from build123d import *

# Parameters (mm, degrees)
SKETCH1_R                      = 27.5
SKETCH1_R_2                    = 8.05
BOSS_EXTRUDE1_DEPTH            = 10
SKETCH1_4_R                    = 3.05
CUT_EXTRUDE1_DEPTH             = 4
CBORE_FOR_M4_SHCS1_D           = 4.1
CBORE_FOR_M4_SHCS1_CBORE_D     = 8
CBORE_FOR_M4_SHCS1_CBORE_DEPTH = 4
CIRPATTERN1_COUNT              = 6
SKETCH1_5_R                    = 9.05
CUT_EXTRUDE2_DEPTH             = 8
BOSS_EXTRUDE2_START            = 8
SKETCH1_6_R                    = 29.5
SKETCH1_6_R_2                  = 27.5
BOSS_EXTRUDE2_DEPTH            = 2
M5X0_8_TAPPED_HOLE1_D          = 4.2
CBORE_FOR_M3_SHCS1_D           = 3.4
CBORE_FOR_M3_SHCS1_CBORE_D     = 6.5
CBORE_FOR_M3_SHCS1_CBORE_DEPTH = 3
CIRPATTERN2_COUNT              = 6
SKETCH9_R                      = 11
CUT_EXTRUDE3_DEPTH             = 4


with BuildPart() as part:
    # Sketch1 → Boss-Extrude1 (new body)
    with BuildSketch(Plane(origin=(0, 0, 0), x_dir=(1, 0, 0), z_dir=(0, 1, 0))):
        with Locations(Location((0, 0, 0), (0, 0, 270))):
            Circle(SKETCH1_R)
        with Locations(Location((0, 0, 0), (0, 0, 270))):
            Circle(SKETCH1_R_2, mode=Mode.SUBTRACT)
    extrude(amount=BOSS_EXTRUDE1_DEPTH)

    # Sketch1<4> → Cut-Extrude1 (cut)
    with BuildSketch(Plane(origin=(0, 0, 0), x_dir=(1, 0, 0), z_dir=(0, 1, 0))):
        with Locations(Location((-20, 0, 0), (0, 0, 270))):
            Circle(SKETCH1_4_R)
        with Locations(Location((-10, 17.320508076, 0), (0, 0, 270))):
            Circle(SKETCH1_4_R)
        with Locations(Location((10, 17.320508076, 0), (0, 0, 270))):
            Circle(SKETCH1_4_R)
        with Locations(Location((20, 0, 0), (0, 0, 270))):
            Circle(SKETCH1_4_R)
        with Locations(Location((10, -17.320508076, 0), (0, 0, 270))):
            Circle(SKETCH1_4_R)
        with Locations(Location((-10, -17.320508076, 0), (0, 0, 270))):
            Circle(SKETCH1_4_R)
    extrude(amount=CUT_EXTRUDE1_DEPTH, mode=Mode.SUBTRACT)

    # CBORE for M4 SHCS1 (through all)
    with Locations(Plane(origin=(0, 10, 0), x_dir=(1, 0, 0), z_dir=(0, 1, 0))):
        with Locations((-20, 0)):
            cbore_for_m4_shcs1 = CounterBoreHole(CBORE_FOR_M4_SHCS1_D / 2, CBORE_FOR_M4_SHCS1_CBORE_D / 2, CBORE_FOR_M4_SHCS1_CBORE_DEPTH)

    # CirPattern1: CBORE for M4 SHCS1 ×6 about axis
    cirpattern1_axis = Axis((0, 0, 0), (0, 1, 0))
    for i in range(1, CIRPATTERN1_COUNT):
        add(cbore_for_m4_shcs1.rotate(cirpattern1_axis, i * 360 / CIRPATTERN1_COUNT), mode=Mode.SUBTRACT)

    # Sketch1<5> → Cut-Extrude2 (cut)
    with BuildSketch(Plane(origin=(0, 0, 0), x_dir=(1, 0, 0), z_dir=(0, 1, 0))):
        with Locations(Location((0, 0, 0), (0, 0, 270))):
            Circle(SKETCH1_5_R)
    extrude(amount=CUT_EXTRUDE2_DEPTH, mode=Mode.SUBTRACT)

    # Sketch1<6> → Boss-Extrude2 (add)
    with BuildSketch(Plane(origin=(0, 0, 0), x_dir=(1, 0, 0), z_dir=(0, 1, 0)).offset(BOSS_EXTRUDE2_START)):
        with Locations(Location((0, 0, 0), (0, 0, 270))):
            Circle(SKETCH1_6_R)
        with Locations(Location((0, 0, 0), (0, 0, 270))):
            Circle(SKETCH1_6_R_2, mode=Mode.SUBTRACT)
    extrude(amount=BOSS_EXTRUDE2_DEPTH)

    # M5x0.8 Tapped Hole1 (through all)
    with Locations(Plane(origin=(0, 10, 0), x_dir=(1, 0, 0), z_dir=(0, 1, 0))):
        with Locations((0, 23)):
            m5x0_8_tapped_hole1 = Hole(M5X0_8_TAPPED_HOLE1_D / 2)

    # CBORE for M3 SHCS1 (through all)
    with Locations(Plane(origin=(0, 10, 0), x_dir=(1, 0, 0), z_dir=(0, 1, 0))):
        with Locations((0, 15)):
            cbore_for_m3_shcs1 = CounterBoreHole(CBORE_FOR_M3_SHCS1_D / 2, CBORE_FOR_M3_SHCS1_CBORE_D / 2, CBORE_FOR_M3_SHCS1_CBORE_DEPTH)

    # CirPattern2: M5x0.8 Tapped Hole1, CBORE for M3 SHCS1 ×6 about axis
    cirpattern2_axis = Axis((0, 0, 0), (0, 1, 0))
    add([m5x0_8_tapped_hole1.rotate(cirpattern2_axis, i * 360 / CIRPATTERN2_COUNT) for i in range(1, CIRPATTERN2_COUNT)], mode=Mode.SUBTRACT)
    add([cbore_for_m3_shcs1.rotate(cirpattern2_axis, i * 360 / CIRPATTERN2_COUNT) for i in range(1, CIRPATTERN2_COUNT)], mode=Mode.SUBTRACT)

    # Sketch9 → Cut-Extrude3 (cut)
    with BuildSketch(Plane.XZ):
        with Locations(Location((0, 0, 0), (0, 0, 270))):
            Circle(SKETCH9_R)
    extrude(amount=-CUT_EXTRUDE3_DEPTH, mode=Mode.SUBTRACT)


solid = part.part
Build history of the part. All positions in model axes, mm. A direction names the side the tool comes from. Coordinates: 2 decimals unless noted, no trailing zeros. Order: outer loops, then holes, each group sorted by start corner. A loop starts at its lowest first (then second) coordinate and runs counter-clockwise, first axis right, second up. Notation, with made-up numbers: (12.5, -4) - (38.5, -4) arc R23 cw to (38.5, 6) - close; hole circle Ø2 at (39, 68.25). An arc over 180 degrees is marked (long way). Write each question's results on one line, items separated by ' | '. Start each with the question number.
Item 1: Band-saw the part on C-C on y = 2. State how many separate pieces and enclosed holes the cut face has, and give its area (3 significant figures).
Item 2: Tool access for faces 1 (the face through (-13.36, 3.45, -9.16)), 2 (the face through (-9, 4, -2)), 3 (the face through (-22, 6, -1)): list every direction of +Z, -Z, +X, -X, +Y, -Y with a clear straight run to the whole face (end or side of a thin tool).
Item 3: Flat gauge pins, fed straight in: pin 1 (5 mm diameter, centred on x = -9.5, z = 18, fed in from -Y); pin 2 (6.5 mm diameter, centred on x = 10, z = 17.32, fed in from +Y); pin 3 (2 mm diameter, centred on x = 17.5, y = 5, fed in from -Z); pin 4 (1.5 mm diameter, centred on x = -5.5, y = 6, fed in from -Z). Where does each tip first touch, or does it go through?
Item 4: Band-saw the part on A-A on z = 23. Write the cut outline in (x, y).
Item 5: Band-saw the part on B-B on x = -20. Write the cut outline in (y, z).
Item 6: Wall check: probe 1 along X at (y, z) = (2.8, 0); probe 2 along Z at (x, y) = (-18.5, 7); probe 3 along Z at (x, y) = (-3, 9). Give the ranges that are in metal, low to high. Write a range as [from, to].
Numbers:
1) separate pieces: 1 | enclosed holes: 19 | area: 1,680 mm^2
2) face 1: +Y, -Y | face 2: -Y | face 3: +Y
3) pin 1: y = 0 | pin 2: y = 6 | pin 3: z = -22 | pin 4: z = -27.09
4) outline: (-18.47, 8) - (-15.07, 8) - (-15.07, 0) - (-2.1, 0) - (-2.1, 10) - (-18.47, 10) - close; (2.1, 0) - (15.07, 0) - (15.07, 8) - (18.47, 8) - (18.47, 10) - (2.1, 10) - close
5) outline: (0, -18.87) - (8, -18.87) - (8, -21.69) - (10, -21.69) - (10, -13.6) - (0, -13.6) - close; (0, -9.4) - (10, -9.4) - (10, -4) - (6, -4) - (6, -2.05) - (4, -2.05) - (4, -3.05) - (0, -3.05) - close; (0, 3.05) - (4, 3.05) - (4, 2.05) - (6, 2.05) - (6, 4) - (10, 4) - (10, 9.4) - (0, 9.4) - close; (0, 13.6) - (10, 13.6) - (10, 21.69) - (8, 21.69) - (8, 18.87) - (0, 18.87) - close
6) probe 1: [-27.5, -23.05], [-16.95, -11], [11, 16.95], [23.05, 27.5] | probe 2: [-20.35, -13.05], [-9.95, -3.71], [3.71, 9.95], [13.05, 20.35] | probe 3: [-29.35, -16.25], [-13.75, -7.47], [7.47, 13.75], [16.25, 29.35]
